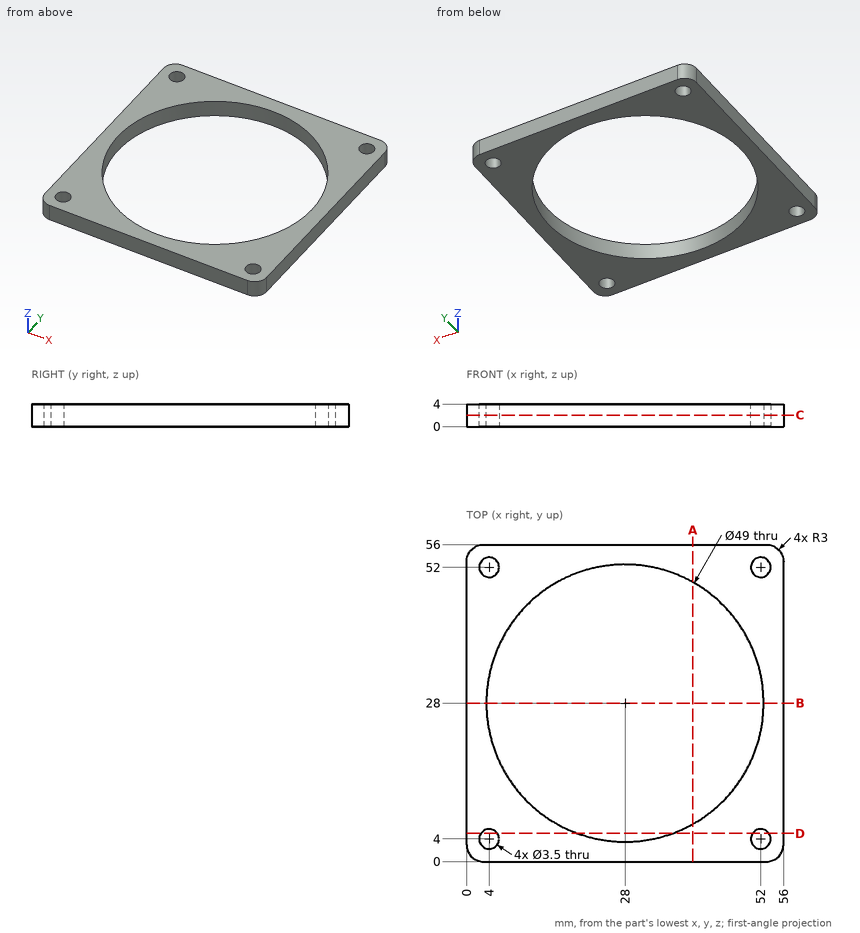
Design review of the part shown in the three views and the two pictorial views. Dimensions are in mm from the part's minimum x, y and z. Give positions to 0.01 mm unless a question says otherwise; leave off trailing zeros. Loops run counter-clockwise (first coordinate to the right, second up) from the corner with the lowest first, then second, coordinate; pieces in that order, holes last. Notation, with made-up numbers: (60.25, 78.5) -> (100.25, 78.5) arc R22 cw to (100.25, 105.5) -> close; hole circle Ø6 at (-23.5, 38). An arc over 180 degrees is marked (long way). Answer as a JSON object with one key per item and string values. Group by question number.
Q1. Take a section at A-A (x = 40). Write out the cut boundary in (y, z), plus the area to 3 significant figures.
Q2. Take a section at B-B (y = 28). Write out the cut boundary in (x, z).
Q3. Take a section at C-C (z = 2.05). Write out the cut boundary in (x, y).
Q4. Wall thickness on line 1 along Y through (x, z) = (50.5, 2.25); line 2 along Y through (x, z) = (27.5, 3.3); line 3 along X through (y, z) = (6, 2.8): over which ranges is each line inside the solid? List them lowest first.
Q5. Take a section at D-D (y = 5). Write out the cut boundary in (x, z).
Q6. Insertion check: pin 1 (2 mm diameter, centred on x = 4, y = 52, fed in from +Z); pin 2 (5.5 mm diameter, centred on x = 52, y = 52, fed in from +Z). Each pin has a flat end and moves straight along its axis. Give the tip position at first contact, or say it passes through.
Answer below:
{
 "1": {"outline": "(0, 0) -> (6.64, 0) -> (6.64, 4) -> (0, 4) -> close; (49.36, 0) -> (56, 0) -> (56, 4) -> (49.36, 4) -> close", "area": "53.1 mm2"},
 "2": {"outline": "(0, 0) -> (3.5, 0) -> (3.5, 4) -> (0, 4) -> close; (52.5, 0) -> (56, 0) -> (56, 4) -> (52.5, 4) -> close"},
 "3": {"outline": "(0, 3) arc R3 ccw to (3, 0) -> (53, 0) arc R3 ccw to (56, 3) -> (56, 53) arc R3 ccw to (53, 56) -> (3, 56) arc R3 ccw to (0, 53) -> close; hole circle Ø3.5 at (4, 4); hole circle Ø3.5 at (4, 52); hole circle Ø49 at (28, 28); hole circle Ø3.5 at (52, 4); hole circle Ø3.5 at (52, 52)"},
 "4": {"line 1": "y = 0 to 3.1, 4.9 to 18.3, 37.7 to 51.1, 52.9 to 56", "line 2": "y = 0 to 3.51, 52.49 to 56", "line 3": "x = 0 to 17.22, 38.78 to 56"},
 "5": {"outline": "(0, 0) -> (2.56, 0) -> (2.56, 4) -> (0, 4) -> close; (5.44, 0) -> (19.56, 0) -> (19.56, 4) -> (5.44, 4) -> close; (36.44, 0) -> (50.56, 0) -> (50.56, 4) -> (36.44, 4) -> close; (53.44, 0) -> (56, 0) -> (56, 4) -> (53.44, 4) -> close"},
 "6": {"pin 1": "passes through", "pin 2": "stops at z = 4"}
}
